Here's how the part is built. I have some questions about the finished solid (model axes, mm). Face numbers are marked on the shaded views. A direction names the side the tool comes from. Coordinates: 2 decimals unless noted, no trailing zeros. Write each loop counter-clockwise with the first axis right and the second up, starting at its lowest first coordinate (ties: lowest second). Pieces come first, ordered by that corner, then holes. Notation, with made-up numbers: (60.5, 57.5) -> (105.5, 57.5) arc R23 ccw to (105.5, 76.5) -> close; hole circle Ø3 at (53, -4). An arc over 180 degrees is marked (long way). Put each result on its own line as item: value.
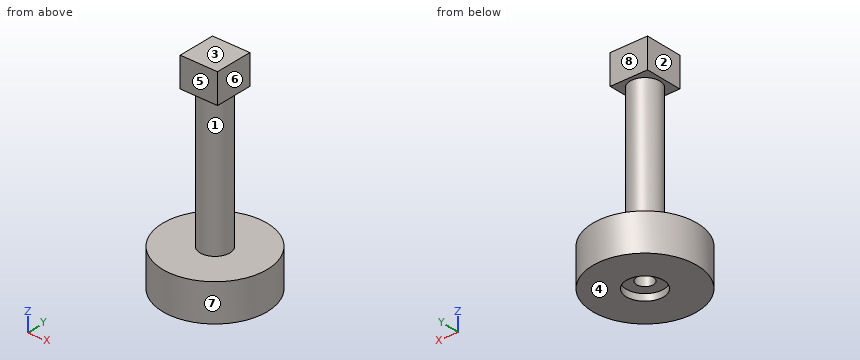
```python
from build123d import *

# Parameters (mm, degrees)
SKETCH1_R           = 14
BOSS_EXTRUDE1_DEPTH = 10
SKETCH2_R           = 2.25
CUT_EXTRUDE1_DEPTH  = 5
SKETCH3_R           = 5
CUT_EXTRUDE2_DEPTH  = 1.8
SKETCH11_R          = 4
BOSS_EXTRUDE2_DEPTH = 37.5
SKETCH12_W          = 10
SKETCH12_H          = 10
BOSS_EXTRUDE3_DEPTH = 8


with BuildPart() as part:
    # Sketch1 → Boss-Extrude1 (new body)
    with BuildSketch(Plane.XY):
        Circle(SKETCH1_R)
    extrude(amount=BOSS_EXTRUDE1_DEPTH)

    # Sketch2 → Cut-Extrude1 (cut)
    with BuildSketch(Plane(origin=(0, 0, 0), x_dir=(-1, 0, 0), z_dir=(0, 0, -1))):
        Circle(SKETCH2_R)
    extrude(amount=-CUT_EXTRUDE1_DEPTH, mode=Mode.SUBTRACT)

    # Sketch3 → Cut-Extrude2 (cut)
    with BuildSketch(Plane(origin=(0, 0, 0), x_dir=(-1, 0, 0), z_dir=(0, 0, -1))):
        Circle(SKETCH3_R)
    extrude(amount=-CUT_EXTRUDE2_DEPTH, mode=Mode.SUBTRACT)

    # Sketch11 → Boss-Extrude2 (add)
    with BuildSketch(Plane.XY.offset(10)):
        Circle(SKETCH11_R)
    extrude(amount=BOSS_EXTRUDE2_DEPTH)

    # Sketch12 → Boss-Extrude3 (add)
    with BuildSketch(Plane.XY.offset(47.5)):
        Rectangle(SKETCH12_W, SKETCH12_H)
    extrude(amount=BOSS_EXTRUDE3_DEPTH)


solid = part.part
```
Item 1: Imagine slicing it at D-D on z = 52.5. Write out the boundary of the cut face in (x, y).
Output:
outline: (-5, -5) -> (5, -5) -> (5, 5) -> (-5, 5) -> close
Item 2: If we mould it in two halves opening along Z, with no side actions, what happens to the marked faces 1, 2, 3 and 4? For each: released by +Z, released by -Z, zero draft, split by the parting line, or undercut.
Output:
face 1: undercut
face 2: zero draft
face 3: released by +Z
face 4: released by -Z
Item 3: For P1, Ø6.5, axis at x = 0, z = 53, coming from the -Y side; P2, Ø1.5, axis at x = -10.5, y = 3.5, coming from the +Z side; P3, Ø9, axis at y = 2.5, z = 51.5, coming from the -X side, each with a flat end and sliding along its axis, tell me the tip position at first contact or that it passes through.
Output:
P1: stops at y = -5
P2: stops at z = 10
P3: stops at x = -5
Item 4: Please list where these lines run through material, in increasing order: line 1 along Y through (x, z) = (0, 1.2); line 2 along Z through (x, y) = (12.75, 0.25); line 3 along Y through (x, z) = (0.5, 8). Write a range as from..to.
Output:
line 1: y = -14..-5, 5..14
line 2: z = 0..10
line 3: y = -13.99..13.99
Item 5: Imagine slicing it at C-C on z = 7. Write out the boundary of the cut face in (x, y), then the cut area to 3 significant figures.
Output:
outline: circle Ø28 at (0, 0)
area: 616 mm²
Item 6: Which directions (+Z, -Z, +X, -X, +Y, -Y) give clear straight access to the entire face, cutting with the end or side of a thin tool? Please do the marked faces 5, 6, 7 and 8.
Output:
face 5: +Z, +X, -X, -Y
face 6: +Z, +X, +Y, -Y
face 7: +Z, -Z
face 8: +Z, +X, -X, +Y
Item 7: Imagine slicing it at A-A on x = 0. Write out the boundary of the cut face in (y, z).
Output:
outline: (-14, 0) -> (-5, 0) -> (-5, 1.8) -> (-2.25, 1.8) -> (-2.25, 5) -> (2.25, 5) -> (2.25, 1.8) -> (5, 1.8) -> (5, 0) -> (14, 0) -> (14, 10) -> (4, 10) -> (4, 47.5) -> (5, 47.5) -> (5, 55.5) -> (-5, 55.5) -> (-5, 47.5) -> (-4, 47.5) -> (-4, 10) -> (-14, 10) -> close
